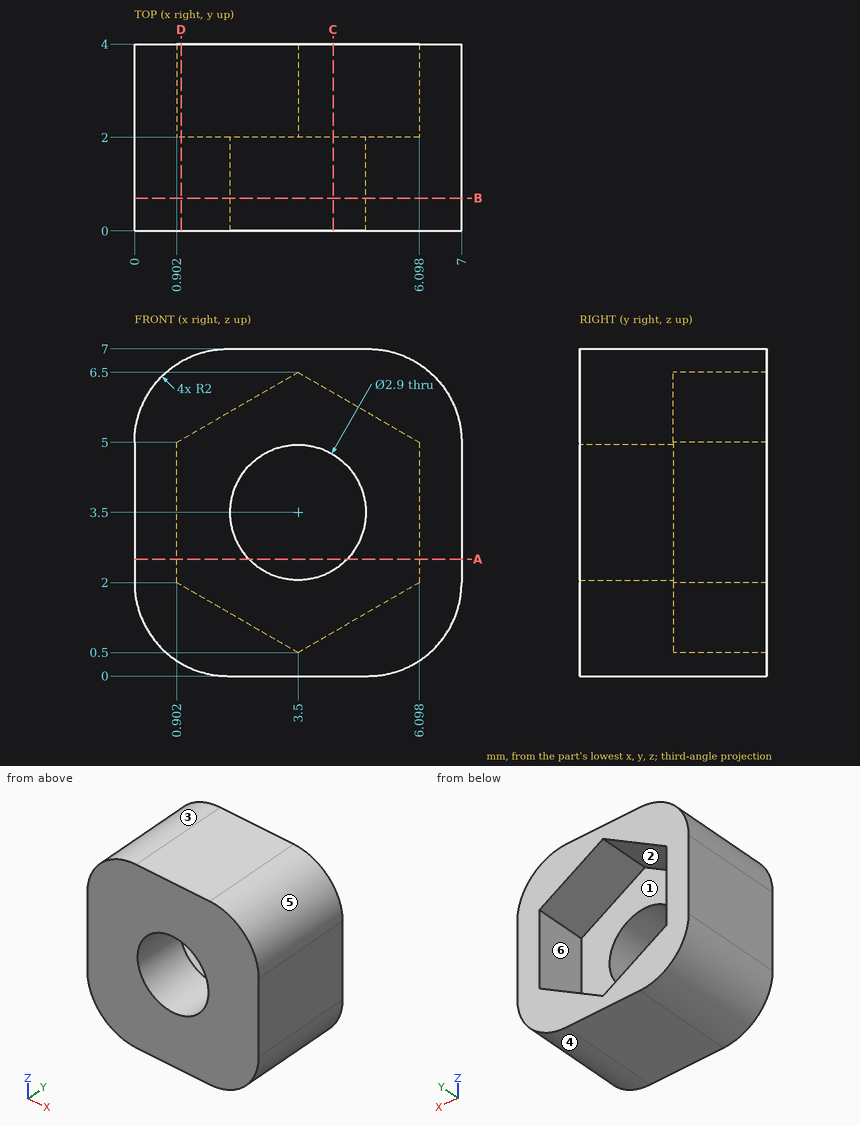
Design review of the part shown in the three views and the two pictorial views. Dimensions are in mm from the part's minimum x, y and z. A direction names the side the tool comes from. Round coordinates to 2 decimals unless told otherwise and drop trailing zeros. Write each loop counter-clockwise with the first axis right and the second up, starting at its lowest first coordinate (ties: lowest second). Pieces come first, ordered by that corner, then holes. Notation, with made-up numbers: M -24.5,49.25 L 10.5,49.25 A26 cw 10.5,78.25 Z; hole C 58.5,-6.5 d11. An arc over 180 degrees is marked long. Use a Markdown table: item, result. Add a question column.
Q1. We need section D-D, the plane x = 1. State the section outline as (y, z) points, plus the area to 3 significant figures.
Q2. We need section C-C, the plane x = 4.25. State the section outline as (y, z) points, plus the area to 3 significant figures.
Q3. We need section B-B, the plane y = 0.7. State the section outline as (x, z) points, plus the area to 3 significant figures.
Q4. We need section A-A, the plane z = 2.5. State the section outline as (x, y) points, plus the area to 3 significant figures.
Q5. To check wall thickness, follow line 1 (X direction, y = 2.55, z = 4); line 2 (X direction, y = 1, z = 3.5); line 3 (Y direction, x = 1, z = 4). State the ranges of each line that lie inside material, in increasing order.
Q6. The part is to be moulded in two halves that separate along X. For the marked faces 1, 2, 3 and 4, say which applies: pulls with the +X half, pulls with the -X half, needs draft (parallel to the pull), parting line crosses it, or undercut.
Q7. Insertion check: pin 1 (1 mm diameter, centred on y = 2.5, z = 4, fed in from -X); pin 2 (1.6 mm diameter, centred on x = 4, z = 2, fed in from +Y); pin 3 (2.5 mm diameter, centred on x = 3.5, z = 3.5, fed in from -Y). Each pin has a flat end and moves straight along its axis. Give the tip position at first contact, or say it passes through.
Q8. Machinability: for the marked faces 5 and 6, which of the approach directions +Z, -Z, +X, -X, +Y, -Y give a long, thin tool a straight path to every point of the face, cutting with its end or side? Answer none if there is none.
Findings below:
| question | item | result |
|---|---|---|
| 1 | outline | M 0,0.27 L 4,0.27 L 4,1.94 L 2,1.94 L 2,5.06 L 4,5.06 L 4,6.73 L 0,6.73 Z |
| 1 | area | 19.6 mm² |
| 2 | outline | M 0,0 L 4,0 L 4,0.93 L 2,0.93 L 2,2.26 L 0,2.26 Z; M 0,4.74 L 2,4.74 L 2,6.07 L 4,6.07 L 4,7 L 0,7 Z |
| 2 | area | 12.8 mm² |
| 3 | outline | M 0,2 A2 ccw 2,0 L 5,0 A2 ccw 7,2 L 7,5 A2 ccw 5,7 L 2,7 A2 ccw 0,5 Z; hole C 3.5,3.5 d2.9 |
| 3 | area | 39.0 mm² |
| 4 | outline | M 0,0 L 2.45,0 L 2.45,2 L 0.9,2 L 0.9,4 L 0,4 Z; M 4.55,0 L 7,0 L 7,4 L 6.1,4 L 6.1,2 L 4.55,2 Z |
| 4 | area | 13.4 mm² |
| 5 | line 1 | x = 0 to 0.9, 6.1 to 7 |
| 5 | line 2 | x = 0 to 2.05, 4.95 to 7 |
| 5 | line 3 | y = 0 to 2 |
| 6 | face 1 | undercut |
| 6 | face 2 | undercut |
| 6 | face 3 | pulls with the -X half |
| 6 | face 4 | pulls with the +X half |
| 7 | pin 1 | stops at x = 0 |
| 7 | pin 2 | stops at y = 2 |
| 7 | pin 3 | passes through |
| 8 | face 5 | +Z, +X, +Y, -Y |
| 8 | face 6 | +Y |
